from build123d import *

# Parameters (mm, degrees)
F2_R     = 3.7933293271
F4_W     = 44.7215028107
F4_H     = 71.540701203
F5_DEPTH = 1.27


# Not quite as in the source:
# - a feature of the source that left no trace in its solid (it failed there, or was rolled back) is left out


with BuildPart() as f3:
    # F3: sweep along a path in F0
    with BuildLine(Plane.XZ) as f3_path:
        Line((-44.6055270731, 57.5704574585), (-44.6055270731, -13.7366456911))
        ThreePointArc((-44.6055270731, -13.7366456911), (-22.3027635366, -36.0394092277), (0, -13.7366456911))
        Line((0, -13.7366456911), (0, 58.4965236485))
    # F2 (on line) → F3 (sweep)
    with BuildSketch(Plane(origin=(0, 0, 57.5704574585), x_dir=(1, 0, 0), z_dir=(0, 0, -1))):
        with Locations((-44.3615987897, 0)):
            Circle(F2_R)
    sweep(path=f3_path.line)

    # F4 (on Front) → F5 (join)
    with BuildSketch(Plane.XZ):
        with Locations((-22.3607514054, 21.9205492176)):
            Rectangle(F4_W, F4_H)
        with BuildLine():
            Line((0, -13.8498013839), (-44.7215028107, -13.8498013839))
            ThreePointArc((-44.7215028107, -13.8498013839), (-22.3607514054, -36.2105527893), (0, -13.8498013839))
        make_face()
    extrude(amount=F5_DEPTH)


solid = f3.part
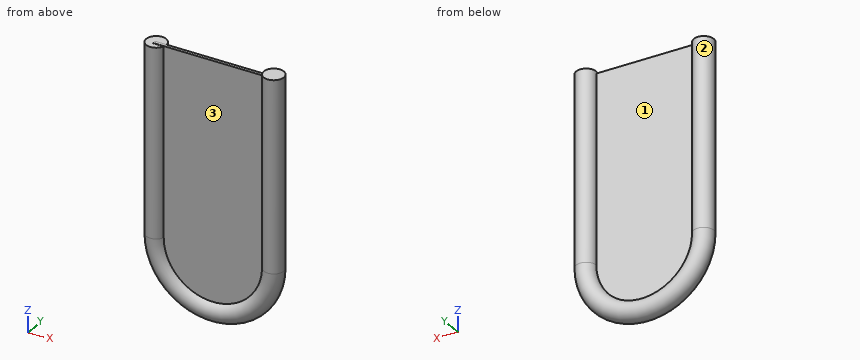
The listing builds one solid part. Answer for the finished solid, in the listing's coordinates (mm). Face numbers are marked on the shaded views. A direction names the side the tool comes from. Give positions to 0.01 mm unless a question says otherwise; leave off trailing zeros. Write each loop counter-clockwise with the first axis right and the second up, starting at its lowest first coordinate (ties: lowest second). Pieces come first, ordered by that corner, then holes.
Item 1: Find the intervals of material crossed by line 1 along Y through (x, z) = (-37.5, 11.5); line 2 along X through (y, z) = (2.5, -10); line 3 along X through (y, z) = (3.25, -8.5), in increasing order.
Item 2: Section A-A, the plane z = -3 is taken. Write down the section's boundary in (x, y).
Item 3: Which of the six approach directions +Z, -Z, +X, -X, +Y, -Y give full straight-line access (tool end or side, diameter ignored) to the marked faces 1, 2 and 3?
Item 4: Flat-ended cylindrical pins translate along their axes: P1, Ø12, axis at x = -22.5, z = 17.5, coming from the +Y side; P2, Ø3, axis at y = 3, z = -3, coming from the +X side; P3, Ø3, axis at y = 1.5, z = 6.5, coming from the +X side; P4, Ø1.4, axis at x = -18.5, y = -0.5, coming from the +Z side. Find the tip coordinate at first contact, or state that the pin passes through.
Completed:
1. line 1: y = -1.27 to 0
1. line 2: x = -47.21 to -41.51, -3.1 to 2.61
1. line 3: x = -46.32 to -42.41, -2.2 to 1.71
2. outline: (-40.79, -1.27) - (-3.82, -1.27) arc R3.79 ccw (long way) to (-4.04, 0) - (-40.57, 0) arc R3.79 ccw (long way) to start
3. face 1: +Z, +Y
3. face 2: +Z
3. face 3: +Z, -Y
4. P1: stops at y = 0
4. P2: stops at x = 3.24
4. P3: stops at x = 3.55
4. P4: stops at z = 57.69
